Check sheet for the drawn part. Datum: minimum x, y, z corner. Units: mm. Coordinates: 2 decimals unless noted, no trailing zeros. Loops run counter-clockwise (first coordinate to the right, second up) from the corner with the lowest first, then second, coordinate; pieces in that order, holes last.
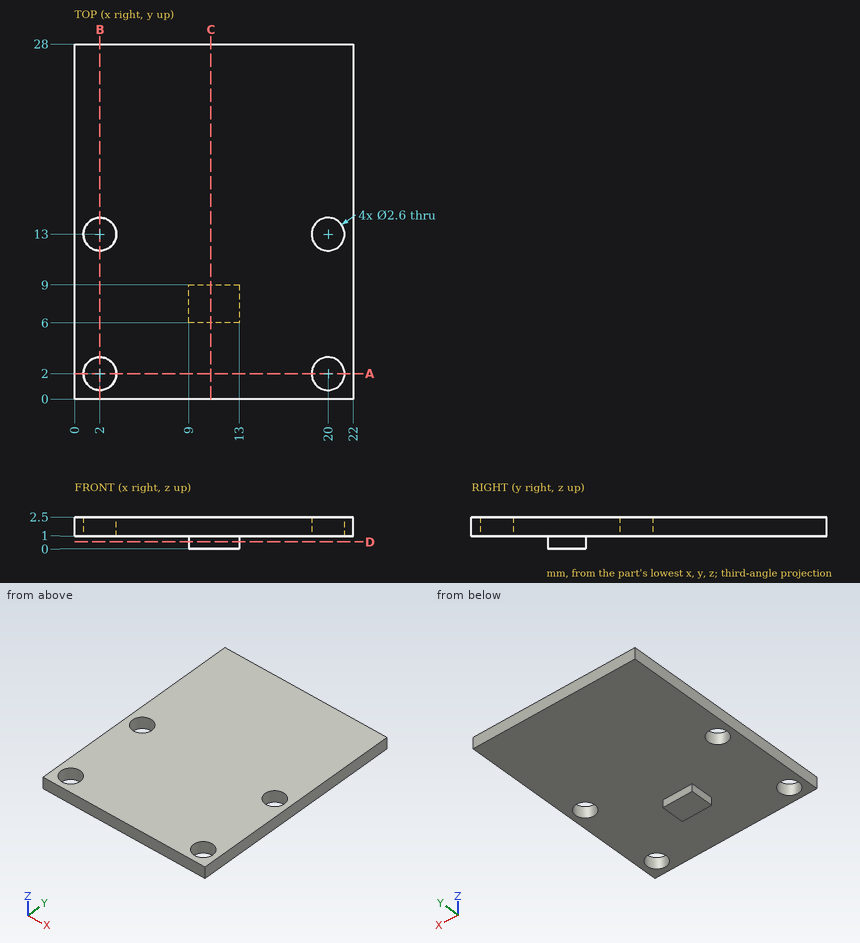
1) Scan lines: line 1 (Y direction, x = 2, z = 1.4); line 2 (Z direction, x = 9.5, y = 17.5); line 3 (X direction, y = 1.5, z = 2.35). Record each from-to range of solid material in increasing order.
Answer sheet:
line 1: y = 0 to 0.7, 3.3 to 11.7, 14.3 to 28
line 2: z = 1 to 2.5
line 3: x = 0 to 0.8, 3.2 to 18.8, 21.2 to 22
2) Depth check by flat-ended pin: pin 1 (6.5 mm diameter, centred on x = 8, y = 13.5, fed in from -Z); pin 2 (1.6 mm diameter, centred on x = 20, y = 13, fed in from -Z); pin 3 (0.8 mm diameter, centred on x = 10.5, z = 0.5, fed in from +Y). Enter the tip coordinate at first touch or a pass-through.
Answer sheet:
pin 1: stops at z = 1
pin 2: passes through
pin 3: stops at y = 9
3) Section check D-D on z = 0.55. Enter the section's corners in (x, y).
Answer sheet:
outline: (9, 6) - (13, 6) - (13, 9) - (9, 9) - close
4) Section check A-A on y = 2. Enter the section's corners in (x, z).
Answer sheet:
outline: (0, 1) - (0.7, 1) - (0.7, 2.5) - (0, 2.5) - close; (3.3, 1) - (18.7, 1) - (18.7, 2.5) - (3.3, 2.5) - close; (21.3, 1) - (22, 1) - (22, 2.5) - (21.3, 2.5) - close
5) Section check B-B on x = 2. Enter the section's corners in (y, z).
Answer sheet:
outline: (0, 1) - (0.7, 1) - (0.7, 2.5) - (0, 2.5) - close; (3.3, 1) - (11.7, 1) - (11.7, 2.5) - (3.3, 2.5) - close; (14.3, 1) - (28, 1) - (28, 2.5) - (14.3, 2.5) - close
6) Section check C-C on x = 10.75. Enter the section's corners in (y, z).
Answer sheet:
outline: (0, 1) - (6, 1) - (6, 0) - (9, 0) - (9, 1) - (28, 1) - (28, 2.5) - (0, 2.5) - close
